```python
from build123d import *

# Parameters (mm, degrees)
BOSS_EXTRUDE1_DEPTH = 20
SKETCH4_R           = 7.5
CUT_EXTRUDE1_DEPTH  = 20
BOSS_EXTRUDE2_DEPTH = 5
BOSS_EXTRUDE3_START = -5
SKETCH9_R           = 5
BOSS_EXTRUDE3_DEPTH = 15


with BuildPart() as part:
    # Sketch2 → Boss-Extrude1 (new body)
    with BuildSketch(Plane.XY):
        with BuildLine():
            Line((-200, 20), (200, 20))
            ThreePointArc((200, 20), (220, 0), (200, -20))
            Line((200, -20), (-200, -20))
            ThreePointArc((-200, -20), (-220, 0), (-200, 20))
        make_face()
    extrude(amount=BOSS_EXTRUDE1_DEPTH)

    # Sketch4 → Cut-Extrude1 (cut)
    with BuildSketch(Plane.XY.offset(20)):
        with Locations((-200, 0)):
            Circle(SKETCH4_R)
        with Locations((200, 0)):
            Circle(SKETCH4_R)
    extrude(amount=-CUT_EXTRUDE1_DEPTH, mode=Mode.SUBTRACT)

    # Sketch8 → Boss-Extrude2 (add)
    with BuildSketch(Plane.XY):
        with BuildLine():
            Line((-150.037555006, -20), (-110.037555006, -20))
            add(Edge.make_bspline(
                [(-150.037555006, -20), (-130.493208153, -80.001537629), (-110.037555006, -20)],
                knots=[0, 0, 0, 1, 1, 1], degree=2))
        make_face()
    boss_extrude2 = extrude(amount=BOSS_EXTRUDE2_DEPTH)

    # Sketch9 → Boss-Extrude3 (add)
    with BuildSketch(Plane.XY.offset(BOSS_EXTRUDE3_START)):
        with Locations((-130, -35)):
            Circle(SKETCH9_R)
    boss_extrude3 = extrude(amount=BOSS_EXTRUDE3_DEPTH)

    # Mirror2: Boss-Extrude2, Boss-Extrude3 across plane
    add(boss_extrude2.mirror(Plane.XY.offset(10)))
    add(boss_extrude3.mirror(Plane.XY.offset(10)))


solid = part.part
```
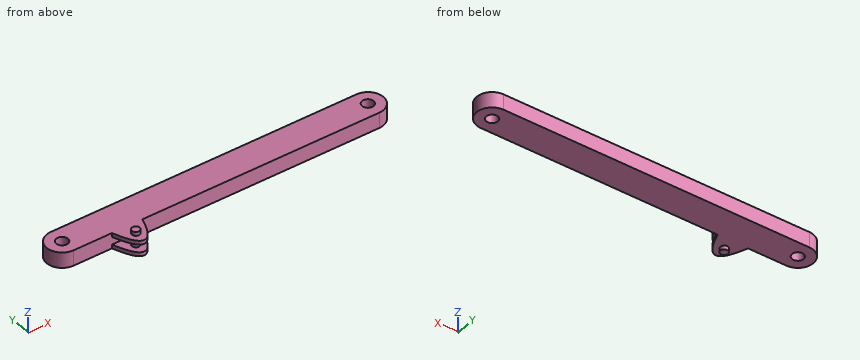
Check sheet for the modelled part. Datum: model origin and axes. Units: mm. Give positions to 0.01 mm unless a question says otherwise; leave off trailing zeros. Order: outer loops, then holes, each group sorted by start corner. A loop starts at its lowest first (then second) coordinate and runs counter-clockwise, first axis right, second up. Notation, with made-up numbers: M 49.25,7 L 106.25,7 A34 cw 106.25,41 Z; hole C 49.25,89 d11. An arc over 180 degrees is marked long. Answer in a Markdown table with one row per item. Add a question column.
Q1. Thickness scan on L1, parallel to Y at x = 200, z = 11; L2, parallel to X at y = 4.5, z = 2.75; L3, parallel to Z at x = -117.5, y = -24. Record the ranges inside material, lowest first.
Q2. Sectioned sample at A-A, the plane y = 0. Record the boundary of the cut face in (x, z), and give its area (3 significant figures).
Q3. Gauge pin test, flat ends, axial feed: pin 1 Ø17 at (x, y) = (-200, 0) entering from -Z; pin 2 Ø5 at (y, z) = (-11, 11) entering from +X; pin 3 Ø8 at (x, y) = (-153, -22) entering from +Z. Record the tip position at first contact, or that the pin passes through.
Q4. Sectioned sample at B-B, the plane x = 45.5. Record the boundary of the cut face in (y, z), and give its area (3 significant figures).
Verdict:
| question | item | result |
|---|---|---|
| 1 | L1 | -20 to -7.5, 7.5 to 20 |
| 1 | L2 | -219.49 to -206, -194 to 194, 206 to 219.49 |
| 1 | L3 | 0 to 5, 15 to 20 |
| 2 | outline | M -220,0 L -207.5,0 L -207.5,20 L -220,20 Z; M -192.5,0 L 192.5,0 L 192.5,20 L -192.5,20 Z; M 207.5,0 L 220,0 L 220,20 L 207.5,20 Z |
| 2 | area | 8,200 mm² |
| 3 | pin 1 | z = 0 |
| 3 | pin 2 | x = 218.1 |
| 3 | pin 3 | z = 20 |
| 4 | outline | M -20,0 L 20,0 L 20,20 L -20,20 Z |
| 4 | area | 800 mm² |
